```python
from build123d import *
from build123d.topology import SkipClean

# Parameters (mm, degrees)
BOSS_EXTRUDE1_DEPTH             = 25
BOSS_EXTRUDE2_REACH             = 65.436
BOSS_EXTRUDE2_DIRECTION_2_DEPTH = 30
SKETCH9_R                       = 2.05
CUT_EXTRUDE3_DEPTH              = 35.1
BOSS_EXTRUDE5_REACH             = 63.632
SKETCH13_R                      = 1.55
CUT_EXTRUDE4_DEPTH              = 88.768186926
SKETCH16_W                      = 50
SKETCH16_H                      = 45
CUT_EXTRUDE5_DEPTH              = 17.55


with BuildPart() as part:
    # Sketch1 → Boss-Extrude1 (new, symmetric)
    with BuildSketch(Plane.XY):
        with BuildLine():
            Line((-17.55, 22.5), (-17.55, 0))
            Line((-17.55, 0), (17.55, 0))
            Line((17.55, 0), (17.55, 22.5))
            Line((17.55, 22.5), (12.55, 22.5))
            ThreePointArc((12.55, 22.5), (0, 9.95), (-12.55, 22.5))
            Line((-12.55, 22.5), (-17.55, 22.5))
        make_face()
    boss_extrude1 = extrude(amount=BOSS_EXTRUDE1_DEPTH, both=True)

    # Boss-Extrude2: up to this face of the body (flat: up to its plane)
    boss_extrude2_end = Plane(part.part.faces().sort_by_distance((17.55, 11.25, 0))[0])
    # Sketch5 → Boss-Extrude2 (add, up to the picked face)
    with BuildSketch(Plane(origin=(26.152881057, 0, 15.099372918), x_dir=(0.500000000000001, 0, -0.8660254037844382), z_dir=(0.8660254037844382, 0, 0.500000000000001)), mode=Mode.PRIVATE) as boss_extrude2_sk1:
        with BuildLine():
            Line((-8.725, 22.5), (-3.775, 22.5))
            ThreePointArc((-3.775, 22.5), (8.775, 9.95), (21.325, 22.5))
            Line((21.325, 22.5), (26.275, 22.5))
            ThreePointArc((26.275, 22.5), (8.775, 5), (-8.725, 22.5))
        make_face()
    boss_extrude2_tool1 = split(extrude(boss_extrude2_sk1.sketch, amount=-BOSS_EXTRUDE2_REACH, mode=Mode.PRIVATE), bisect_by=boss_extrude2_end, keep=Keep.BOTH, mode=Mode.PRIVATE)
    boss_extrude2 = boss_extrude2_tool1.solids().sort_by(Axis((23.027881, 22.108688, 20.512032), (-0.8660254037844382, 0, -0.500000000000001)))[0]
    add(boss_extrude2)

    # Sketch5 → Boss-Extrude2 direction 2 (add)
    with BuildSketch(Plane(origin=(26.152881057, 0, 15.099372918), x_dir=(0.500000000000001, 0, -0.8660254037844382), z_dir=(0.8660254037844382, 0, 0.500000000000001))):
        with BuildLine():
            Line((-8.725, 22.5), (-3.775, 22.5))
            ThreePointArc((-3.775, 22.5), (8.775, 9.95), (21.325, 22.5))
            Line((21.325, 22.5), (26.275, 22.5))
            ThreePointArc((26.275, 22.5), (8.775, 5), (-8.725, 22.5))
        make_face()
    boss_extrude2_direction_2 = extrude(amount=BOSS_EXTRUDE2_DIRECTION_2_DEPTH)

    # Sketch9 → Cut-Extrude3 (cut)
    with BuildSketch(Plane.ZY.offset(17.55)):
        with Locations((-18, 5)):
            Circle(SKETCH9_R)
        with Locations((18, 5)):
            Circle(SKETCH9_R)
    cut_extrude3 = extrude(amount=-CUT_EXTRUDE3_DEPTH, mode=Mode.SUBTRACT)

    # Boss-Extrude5: up to this face of the body (flat: up to its plane)
    boss_extrude5_end = Plane(part.part.faces().sort_by_distance((17.55, 17.173614571, 0))[0])
    # Sketch12 → Boss-Extrude5 (add, up to the picked face)
    with BuildSketch(Plane(origin=(22.035576211, 0, 12.722245857), x_dir=(0.4999999999999999, 0, -0.8660254037844388), z_dir=(0.8660254037844388, 0, 0.4999999999999999)), mode=Mode.PRIVATE) as boss_extrude5_sk1:
        with BuildLine():
            Line((-3.775, 22.5), (21.325, 22.5))
            ThreePointArc((21.325, 22.5), (8.775, 9.95), (-3.775, 22.5))
        make_face()
    boss_extrude5_tool1 = split(extrude(boss_extrude5_sk1.sketch, amount=-BOSS_EXTRUDE5_REACH, mode=Mode.PRIVATE), bisect_by=boss_extrude5_end, keep=Keep.BOTH, mode=Mode.PRIVATE)
    boss_extrude5 = boss_extrude5_tool1.solids().sort_by(Axis((26.423076, 17.173615, 5.122873), (-0.8660254037844388, 0, -0.4999999999999999)))[0]
    add(boss_extrude5)


with BuildPart() as mirror1_1:
    # Mirror1: Boss-Extrude1, Boss-Extrude2, Boss-Extrude2 direction 2 across plane
    add(boss_extrude1.mirror(Plane(origin=(17.55, 22.5, 25), x_dir=(0, 0, 1), z_dir=(0, -1, 0))))
    add(boss_extrude2.mirror(Plane(origin=(17.55, 22.5, 25), x_dir=(0, 0, 1), z_dir=(0, -1, 0))))
    add(boss_extrude2_direction_2.mirror(Plane(origin=(17.55, 22.5, 25), x_dir=(0, 0, 1), z_dir=(0, -1, 0))))

    # Mirror1 2: Cut-Extrude3 across plane
    add(cut_extrude3.mirror(Plane(origin=(17.55, 22.5, 25), x_dir=(0, 0, 1), z_dir=(0, -1, 0))), mode=Mode.SUBTRACT)


with BuildPart() as mirror1_3_1:
    # Mirror1 3: Boss-Extrude5 across plane
    add(boss_extrude5.mirror(Plane(origin=(17.55, 22.5, 25), x_dir=(0, 0, 1), z_dir=(0, -1, 0))))


with BuildPart() as part_1:
    add(part.part)

    # Mirror1 united with what the copies touc: union Mirror1_1, Mirror1 3_1
    add(mirror1_1.part)
    add(mirror1_3_1.part)

    # Sketch13 → Cut-Extrude4 (cut, through all)
    with SkipClean():  # the faces are left unmerged after this step: merging them gives an invalid solid
        with BuildSketch(Plane(origin=(0, 0, 0), x_dir=(1, 0, 0), z_dir=(0, 1, 0))):
            with Locations(Location((43.530762114, -15, 0), (0, 0, 90))):
                Circle(SKETCH13_R)
        extrude(amount=CUT_EXTRUDE4_DEPTH, mode=Mode.SUBTRACT)

    # Sketch16 → Cut-Extrude5 (cut)
    with BuildSketch(Plane(origin=(0, 0, 0), x_dir=(0, 0, -1), z_dir=(1, 0, 0))):
        with Locations((0, 22.5)):
            Rectangle(SKETCH16_W, SKETCH16_H)
    extrude(amount=-CUT_EXTRUDE5_DEPTH, mode=Mode.SUBTRACT)


solid = part_1.part
```
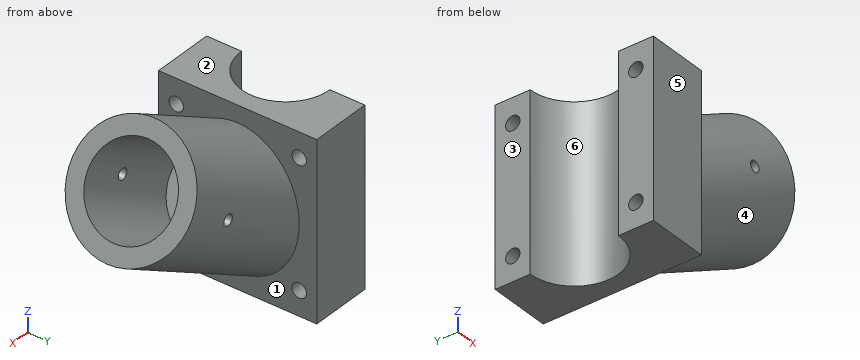
Model file for the job. Use its own axes, mm. Face numbers are marked on the shaded views. A direction names the side the tool comes from. Coordinates: 2 decimals unless noted, no trailing zeros. Loops run counter-clockwise (first coordinate to the right, second up) from the corner with the lowest first, then second, coordinate; pieces in that order, holes last. Notation, with made-up numbers: (75, 21.25) -> (124, 21.25) arc R25 cw to (124, 58.25) -> close; hole circle Ø2 at (-32.75, -31). An arc over 180 degrees is marked (long way). Answer as a JSON object with one key per item and string values.
Q1. 3-axis set-ups, long thin cutter, end or side, ignore diameter. For the marked faces 1, 2 and 3: which of +Z, -Z, +X, -X, +Y, -Y reach the whole face in a straight line?
Report:
{"face 1": "none", "face 2": "+Z, -X, +Y, -Y", "face 3": "+Z, -Z, -X, +Y, -Y"}
Q2. Flat gauge pins, fed straight in: P1, Ø6, axis at y = 15, z = 1, coming from the +X side; P2, Ø5, axis at x = 53.5, z = 26, coming from the +Y side; P3, Ø4, axis at x = 43.53, z = 15, coming from the +Y side; P4, Ø10, axis at y = 12, z = 27.5, coming from the -X side. Where does each tip first touch, or does it go through?
Report:
{"P1": "stops at x = 56.7", "P2": "stops at y = 39.88", "P3": "stops at y = 40", "P4": "stops at x = 0"}
Q3. Cut at C-C (y = 34). List the corners of the cut face in (x, z), and give its area (3 significant figures).
Report:
{"outline": "(5.03, -25) -> (17.55, -25) -> (17.55, -15.23) -> (63.12, 11.08) -> (59.03, 18.15) -> (28.94, 0.77) -> (23.91, 9.47) -> (54.01, 26.85) -> (49.93, 33.92) -> (17.55, 15.23) -> (17.55, 25) -> (5.03, 25) -> close", "area": "1,460 mm2"}
Q4. Pull direction Y, two halves, no side cores. Call the marked faces 4, 5 and 6: released by +Y, released by -Y, zero draft, split by the parting line, or undercut.
Report:
{"face 4": "split by the parting line", "face 5": "released by -Y", "face 6": "undercut"}
Q5. Probe probe 1 along Y at (x, z) = (7.25, -18); probe 2 along Z at (x, y) = (17.5, 9); probe 3 along Y at (x, z) = (14, 19). List the from-to ranges inside material, lowest first.
Report:
{"probe 1": "y = 0 to 2.95, 7.05 to 12.26, 32.74 to 37.95, 42.05 to 45", "probe 2": "z = -25 to 25", "probe 3": "y = 0 to 3.21, 6.79 to 38.21, 41.79 to 45"}
Q6. Cut at A-A (x = 15). List the corners of the cut face in (y, z), and give its area (3 significant figures).
Report:
{"outline": "(0, -25) -> (45, -25) -> (45, 25) -> (0, 25) -> close; hole circle Ø4.1 at (5, -18); hole circle Ø4.1 at (5, 18); hole circle Ø4.1 at (40, -18); hole circle Ø4.1 at (40, 18)", "area": "2,200 mm2"}
Q7. Cut at B-B (y = 41). List the corners of the cut face in (x, z).
Report:
{"outline": "(0, -25) -> (17.55, -25) -> (17.55, -19.79) -> (0, -19.79) -> close; (0, -16.21) -> (17.55, -16.21) -> (17.55, 16.21) -> (0, 16.21) -> close; (0, 19.79) -> (17.55, 19.79) -> (17.55, 25) -> (0, 25) -> close"}
Q8. Cut at D-D (z = -18). State how many separate pieces and enclosed holes the cut face has, and give its area (3 significant figures).
Report:
{"separate pieces": "3", "enclosed holes": "0", "area": "439 mm2"}
